```python
from build123d import *

# Parameters (mm, degrees)
SKETCH_R      = 22.5
PAD_DEPTH     = 2
SKETCH001_R   = 22.5
SKETCH001_R_2 = 20.5
PAD001_DEPTH  = 10
SKETCH002_R   = 22.5
SKETCH002_R_2 = 19
PAD002_DEPTH  = 8
SKETCH003_W   = 5
SKETCH003_H   = 20
POCKET_DEPTH  = 22.501


with BuildPart() as part:
    # Sketch → Pad (new body)
    with BuildSketch(Plane.XY):
        Circle(SKETCH_R)
    extrude(amount=PAD_DEPTH)

    # Sketch001 → Pad001 (join)
    with BuildSketch(Plane.XY):
        Circle(SKETCH001_R)
        Circle(SKETCH001_R_2, mode=Mode.SUBTRACT)
    extrude(amount=PAD001_DEPTH)

    # Sketch002 → Pad002 (join)
    with BuildSketch(Plane.XY):
        Circle(SKETCH002_R)
        Circle(SKETCH002_R_2, mode=Mode.SUBTRACT)
    extrude(amount=PAD002_DEPTH)

    # Sketch003 → Pocket (cut, through all)
    with BuildSketch(Plane.XZ):
        with Locations((0, 15)):
            Rectangle(SKETCH003_W, SKETCH003_H)
    extrude(amount=-POCKET_DEPTH, mode=Mode.SUBTRACT)


solid = part.part
```
The listing builds one solid part. Answer for the finished solid, in the listing's coordinates (mm). A direction names the side the tool comes from. Give positions to 0.01 mm unless a question says otherwise; leave off trailing zeros. Order: outer loops, then holes, each group sorted by start corner. A loop starts at its lowest first (then second) coordinate and runs counter-clockwise, first axis right, second up.
Item 1: For a pull along Y with two mould halves and no side action, classify faces 4 (the face through (-9, -17, 8)), 5 (the face through (10.382, -19.961, 4.93)), 6 (the face through (-2.5, 21, 7)) as pulls with the +Y half, pulls with the -Y half, needs draft (parallel to the pull), parting line crosses it, or undercut.
From the geometry:
face 4: undercut
face 5: parting line crosses it
face 6: needs draft
Item 2: The part is cut by section D-D, the plane y = -10. Give the vertices of the cut face in (x, z), and give its area (3 significant figures).
From the geometry:
outline: (-20.16, 0) - (20.16, 0) - (20.16, 10) - (17.9, 10) - (17.9, 8) - (16.16, 8) - (16.16, 2) - (-16.16, 2) - (-16.16, 8) - (-17.9, 8) - (-17.9, 10) - (-20.16, 10) - close
area: 138 mm2
Item 3: Find the intervals of material crossed by probe 1 along X at (y, z) = (0, 8.85); probe 2 along Y at (x, z) = (0, 4.3); probe 3 along Z at (x, y) = (-8, 15.5), in increasing order.
From the geometry:
probe 1: x = -22.5 to -20.5, 20.5 to 22.5
probe 2: y = -22.5 to -19, 19 to 22.5
probe 3: z = 0 to 2
Item 4: Given pin 1 Ø1.8 at (y, z) = (20.5, 6.5) entering from +X; pin 2 Ø1.1 at (x, y) = (1, 21.5) entering from +Z; pin 3 Ø2 at (x, y) = (-9.5, -11) entering from -Z; pin 4 Ø19 at (x, y) = (5, 9) entering from +Z, each flat-ended and moving along its own axis, determine where each tip first touches the part or whether it passes through.
From the geometry:
pin 1: stops at x = 11.05
pin 2: stops at z = 5
pin 3: stops at z = 0
pin 4: stops at z = 8
Item 5: The part is cut by section B-B, the plane y = 0. Give the vertices of the cut face in (x, z), and give its area (3 significant figures).
From the geometry:
outline: (-22.5, 0) - (22.5, 0) - (22.5, 10) - (20.5, 10) - (20.5, 8) - (19, 8) - (19, 2) - (-19, 2) - (-19, 8) - (-20.5, 8) - (-20.5, 10) - (-22.5, 10) - close
area: 140 mm2
Item 6: Which of the six approach directions +Z, -Z, +X, -X, +Y, -Y give full straight-line access (tool end or side, diameter ignored) to faces 1 (the face through (2.5, 21, 7)), 2 (the face through (0, 0, 0)), 3 (the face through (-4.119, -18.548, 4.958))?
From the geometry:
face 1: +Z, +Y
face 2: -Z, +X, -X, +Y, -Y
face 3: +Z
Item 7: The part is cut by section C-C, the plane z = 9. Give the vertices of the cut face in (x, y).
From the geometry:
outline: (-2.5, 20.35) - (-2.5, 22.36) arc R22.5 ccw (long way) to (2.5, 22.36) - (2.5, 20.35) arc R20.5 cw (long way) to start
Item 8: The part is cut by section A-A, the plane x = 0. Give the vertices of the cut face in (y, z).
From the geometry:
outline: (-22.5, 0) - (22.5, 0) - (22.5, 5) - (19, 5) - (19, 2) - (-19, 2) - (-19, 8) - (-20.5, 8) - (-20.5, 10) - (-22.5, 10) - close
